Autodesk Inventor part; units mm, degrees
ref_plane "YZ Plane" through (0, 0, 0) normal (1, 0, 0) x (0, 1, 0)
ref_plane "XZ Plane" through (0, 0, 0) normal (0, 1, 0) x (-1, 0, 0)
ref_plane "XY Plane" through (0, 0, 0) normal (0, 0, 1) x (1, 0, 0)
sketch "Эскиз1" plane through (0, 0, 0) normal (0, 1, 0) x (-1, 0, 0)
  line L0 (-19, 27.5) -> (19, 27.5)
  line L1 (19, 27.5) -> (19, -27.5)
  line L2 (19, -27.5) -> (-19, -27.5)
  line L3 (-19, -27.5) -> (-19, 27.5)
  line L4 (-19, 27.5) -> (19, -27.5) construction
  line L5 (19, 27.5) -> (-19, -27.5) construction
  point P0 (0, 0)
  dimension "d10" = 55
  dimension "d11" = 38
extrude "Выдавливание1" add sketch "Эскиз1" along normal blind 2
sketch "Эскиз2" plane through (0, 2, 0) normal (0, 1, 0) x (1, 0, 0)
  line L0 (7, -18.55) -> (19, -18.55)
  line L1 (19, -18.55) -> (19, -11.55)
  line L2 (19, -11.55) -> (7, -11.55)
  line L3 (7, -11.55) -> (7, -18.55)
  line L4 (7, -18.55) -> (19, -11.55) construction
  line L5 (19, -18.55) -> (7, -11.55) construction
  line L6 (7, 11.55) -> (19, 11.55)
  line L7 (19, 11.55) -> (19, 18.55)
  line L8 (19, 18.55) -> (7, 18.55)
  line L9 (7, 18.55) -> (7, 11.55)
  line L10 (7, 11.55) -> (19, 18.55) construction
  line L11 (19, 11.55) -> (7, 18.55) construction
  line L12 (19, -27.5) -> (19, 27.5)
  line L13 (-19, 27.5) -> (-19, -27.5)
  line L14 (-19, 0) -> (19, 0)
  point P0 (0, 0)
  point P1 (13, -15.05)
  point P2 (13, 15.05)
  point P3 (0, 0)
  dimension "d2" = 12
  dimension "d3" = 7
  dimension "d4" = 12
  dimension "d5" = 7
  dimension "d12" = 0
  dimension "d15" = 0
  dimension "d25" = 11.55
  dimension "d26" = 11.55
extrude "Выдавливание2" add sketch "Эскиз2" along normal blind 14
sketch "Эскиз4" plane through (0, 2, 0) normal (0, 1, 0) x (1, 0, 0)
  circle A0 centre (15, 7.55) radius 1.6
  circle A1 centre (11, -7.55) radius 1.6
  line L0 (7, -11.55) -> (7, -18.55)
  line L1 (7, 11.55) -> (19, 11.55)
  line L2 (19, -11.55) -> (7, -11.55)
  point P0 (0, 0)
  dimension "d17" = 3.2
  dimension "d18" = 3.2
  dimension "d20" = 4
  dimension "d21" = 4
  dimension "d22" = 4
extrude "Выдавливание3" cut sketch "Эскиз4" against normal blind 14
sketch "Эскиз5" plane through (19, 2, 18.55) normal (1, 0, 0) x (0, 0, 1)
  circle A0 centre (-32.3, -3.5) radius 1.25
  circle A1 centre (-32.3, -10.5) radius 1.25
  circle A2 centre (-4.8, -10.5) radius 1.25
  circle A3 centre (-4.8, -3.5) radius 1.25
  line L0 (-4.8, -10.5) -> (-32.3, -10.5) construction
  line L1 (-32.3, -10.5) -> (-32.3, -3.5) construction
  line L2 (-32.3, -3.5) -> (-4.8, -3.5) construction
  line L3 (-4.8, -3.5) -> (-4.8, -10.5) construction
  line L4 (0, 0) -> (0, -14) construction
  line L5 (-37.1, 0) -> (-37.1, -14) construction
  line L6 (0, 0) -> (-37.1, 0) construction
  line L7 (-37.1, 0) -> (-37.1, -14) construction
  line L8 (-37.1, -14) -> (0, -14) construction
  line L9 (0, -14) -> (0, 0) construction
  line L10 (-18.55, -14) -> (-18.55, 0) construction
  line L11 (-46.05, 0) -> (8.95, 0) construction
  line L12 (-18.55, -3.5) -> (-18.55, -10.5) construction
  point P0 (-18.55, -7)
  dimension "d51" = 27.5
  dimension "d52" = 7
  dimension "d55" = 2.5
  dimension "d56" = 2.5
extrude "Выдавливание4" cut sketch "Эскиз5" against normal blind 14
sketch "Эскиз6" plane through (0, 2, 0) normal (0, 1, 0) x (1, 0, 0)
  circle A0 centre (-12, -24.5) radius 1.6
  circle A1 centre (-12, 23.5) radius 1.6
  circle A2 centre (13.5, -24.5) radius 1.6
  circle A3 centre (13.5, 23.5) radius 1.6
  point P0 (0, 0)
extrude "Выдавливание5" cut sketch "Эскиз6" against normal blind 10
sketch "Эскиз7" plane through (7, 2, 18.55) normal (0, 0, 1) x (1, 0, 0)
  line L0 (12, 14) -> (0, 14)
  line L1 (6, 14) -> (6, -2) construction
  line L2 (12, -2) -> (-26, -2)
  line L3 (0, 0) -> (0, 14)
  line L4 (0, 7) -> (12, 7) construction
  line L5 (12, 0) -> (12, 14)
  line L6 (12, 4.75) -> (12, 2.25)
  line L7 (0, 9.5) -> (12, 9.5)
  line L8 (6.8, 7.45) -> (5.2, 7.45)
  line L9 (5.2, 7.45) -> (5.2, 11.55)
  line L10 (5.2, 11.55) -> (6.8, 11.55)
  line L11 (6.8, 11.55) -> (6.8, 7.45)
  line L12 (6.8, 7.45) -> (5.2, 11.55) construction
  line L13 (5.2, 7.45) -> (6.8, 11.55) construction
  point P0 (-7, -2)
  point P1 (0, 8.25)
  point P2 (0, 10.75)
  point P3 (6, 9.5)
  dimension "d31" = 4.5
  dimension "d32" = 1.6
  dimension "d33" = 4.1
extrude "Выдавливание6" cut sketch "Эскиз7" against normal blind 12 contours L11 L8 L9 L7 | L7 L9 L10 L11
mirror "Зеркальное отражение1" about plane through (0, 0, 0) normal (0, 0, 1) of "Выдавливание6"
sketch "Эскиз8" plane through (-19, 0, -27.5) normal (-1, 0, 0) x (0, 0, 1)
  line L0 (0, 0) -> (16, 0)
  line L1 (16, 0) -> (16, 14)
  line L2 (16, 14) -> (0, 14)
  line L3 (0, 14) -> (0, 0)
  point P0 (27.5, 0)
  dimension "d38" = 16
  dimension "d39" = 14
extrude "Выдавливание7" add sketch "Эскиз8" along normal blind 2
sketch "Эскиз9" plane through (-21, 0, -27.5) normal (-1, 0, 0) x (0, 0, 1)
  line L0 (0, 14) -> (0, 0) construction
  line L1 (0, 10) -> (16, 10) construction
  line L2 (16, 0) -> (16, 14) construction
  line L3 (16, 14) -> (0, 14) construction
  circle A0 centre (3.5886, 10) radius 1.6
  circle A1 centre (11.5886, 10) radius 1.6
  line L4 (3.5886, 10) -> (11.5886, 10)
  line L5 (8, 14) -> (8, 2)
  point P0 (27.5, 0)
  point P1 (0, 12)
  point P2 (16, 12)
  point P3 (14, 14)
  point P4 (2, 14)
  dimension "d43" = 4
  dimension "d44" = 3.2
  dimension "d45" = 3.2
  dimension "d46" = 8
extrude "Выдавливание8" cut sketch "Эскиз9" against normal blind 2
fillet "Сопряжение2" radius 2 1 edges at (-19, 2, -19.5)
fillet "Сопряжение3" radius 1 2 edges at (-20, 14, -27.5) (-20, 14, -11.5)
properties part number "креп_сервы"
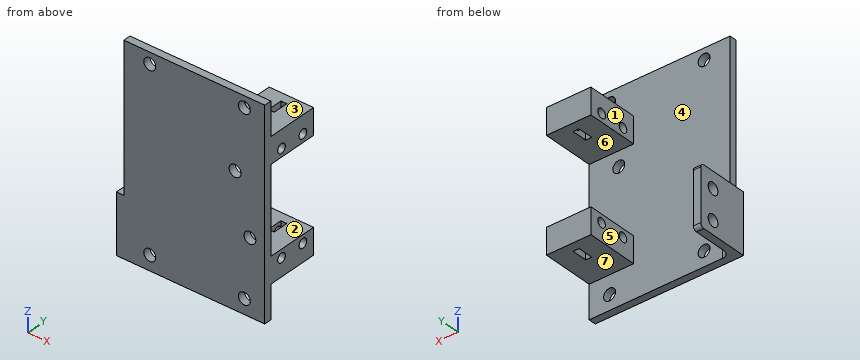
CAD build for the part. Positions are in the model's coordinates, mm. Face numbers are marked on the shaded views. A direction names the side the tool comes from. Give positions to 0.01 mm unless a question says otherwise; leave off trailing zeros. Order: outer loops, then holes, each group sorted by start corner. A loop starts at its lowest first (then second) coordinate and runs counter-clockwise, first axis right, second up. Notation, with made-up numbers: (-22, 50) - (30, 50) arc R15 ccw to (30, 56) - close; hole circle Ø9 at (71.5, -15). An arc over 180 degrees is marked (long way). Write each question's results on one line, items separated by ' | '.
1. Saw through at C-C on z = 24.5. List the corners of the cut face in (x, y).
Calculated:
outline: (-19, 0) - (-13.6, 0) - (-13.6, 2) - (-19, 2) - close; (-10.4, 0) - (11.9, 0) - (11.9, 2) - (-10.4, 2) - close; (15.1, 0) - (19, 0) - (19, 2) - (15.1, 2) - close
2. Probe L1, parallel to X at y = 1.5, z = -23.5; L2, parallel to Z at x = 11.5, y = 12.5; L3, parallel to Z at x = -12, y = 0.7. List the from-to ranges inside material, lowest first. Write a range as from..to.
Calculated:
L1: x = -21..-13.6, -10.4..11.9, 15.1..19 | L2: z = -18.55..-15, -12.5..-11.55, 11.55..12.5, 15..18.55 | L3: z = -27.5..-25.1, -21.9..22.9, 26.1..27.5
3. Saw through at A-A on x = 11. List the corners of the cut face in (y, z), and give its area (3 significant figures).
Calculated:
outline: (0, -27.5) - (2, -27.5) - (2, -18.55) - (16, -18.55) - (16, -11.55) - (2, -11.55) - (2, 5.95) - (0, 5.95) - close; (0, 9.15) - (2, 9.15) - (2, 11.55) - (16, 11.55) - (16, 18.55) - (2, 18.55) - (2, 27.5) - (0, 27.5) - close; hole circle Ø2.5 at (5.5, -13.75); hole circle Ø2.5 at (5.5, 13.75); hole circle Ø2.5 at (12.5, -13.75); hole circle Ø2.5 at (12.5, 13.75) | area: 280 mm2
4. Pin check, flat tips, straight feed: pin 1 (2 mm diameter, centred on x = -2, z = 19.5, fed in from +Y); pin 2 (1 mm diameter, centred on x = 7.5, y = 11.5, fed in from -Z); pin 3 (5 mm diameter, centred on y = 10, z = -23.91, fed in from +X); pin 4 (2 mm diameter, centred on x = -2.5, y = 3.5, fed in from +Z). Stop position of each tip, or through.
Calculated:
pin 1: stops at y = 2 | pin 2: stops at z = -18.55 | pin 3: stops at x = -19 | pin 4: passes through
5. 3-axis set-ups, long thin cutter, end or side, ignore diameter. For the marked faces 1, 2 and 3: which of +Z, -Z, +X, -X, +Y, -Y reach the whole face in a straight line?
Calculated:
face 1: +Z, -Z, -X, +Y | face 2: +X, +Y | face 3: +Z, +X, -X, +Y
6. Saw through at D-D on z = 13.75. List the corners of the cut face in (x, y), and give its area (3 significant figures).
Calculated:
outline: (-19, 0) - (19, 0) - (19, 4.25) - (7, 4.25) - (7, 2) - (-19, 2) - close; (7, 6.75) - (19, 6.75) - (19, 11.25) - (13.8, 11.25) - (13.8, 9.45) - (12.2, 9.45) - (12.2, 11.25) - (7, 11.25) - close; (7, 13.75) - (19, 13.75) - (19, 16) - (7, 16) - close | area: 181 mm2
7. Saw through at B-B on z = 7.55. List the corners of the cut face in (x, y).
Calculated:
outline: (-19, 0) - (9.4, 0) - (9.4, 2) - (-19, 2) - close; (12.6, 0) - (19, 0) - (19, 2) - (12.6, 2) - close
8. Pull direction Z, two halves, no side cores. Call the marked faces 4, 5, 6 and 7: released by +Z, released by -Z, zero draft, split by the parting line, or undercut.
Calculated:
face 4: undercut | face 5: zero draft | face 6: undercut | face 7: released by -Z
